from build123d import *

# Parameters (mm, degrees)
F0_W     = 35.25
F0_H     = 22.25
F1_DEPTH = 10
F2_R     = 1


with BuildPart() as f1:
    # F0 (on Top) → F1 (new body)
    with BuildSketch(Plane.XY):
        with BuildLine():
            Line((21, -9.464824), (21, 9.464824))
            ThreePointArc((21, 9.464824), (19.853951, 12.650269), (16.941176, 14.375444))
            ThreePointArc((16.941176, 14.375444), (0, 15.984287), (-16.941176, 14.375444))
            ThreePointArc((-16.941176, 14.375444), (-19.853951, 12.650269), (-21, 9.464824))
            Line((-21, 9.464824), (-21, -11.101853))
            ThreePointArc((-21, -11.101853), (-20.330458, -12.991023), (-18.62069, -14.036941))
            ThreePointArc((-18.62069, -14.036941), (-0.856643, -15.98021), (16.941176, -14.375444))
            ThreePointArc((16.941176, -14.375444), (19.853951, -12.650269), (21, -9.464824))
        make_face()
        Rectangle(F0_W, F0_H, mode=Mode.SUBTRACT)
    extrude(amount=F1_DEPTH)

    # F2
    f2_edges = [f1.edges().sort_by_distance(p)[0] for p in [
        (19.853951, 12.650269, 10),
        (19.853951, 12.650269, 0),
    ]]
    fillet(f2_edges, radius=F2_R)


solid = f1.part
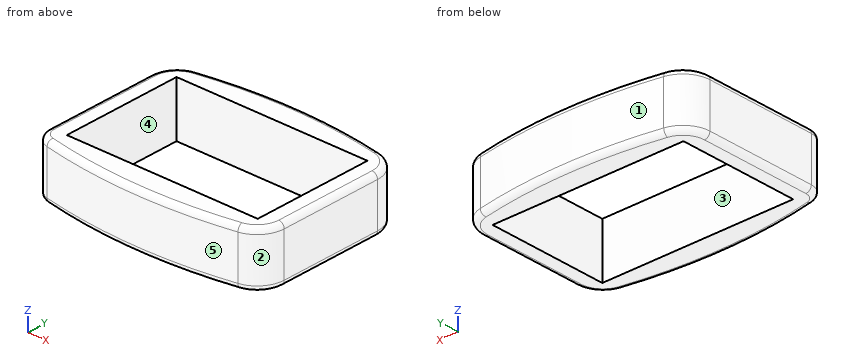
Check sheet for the modelled part. Datum: model origin and axes. Units: mm. Face numbers are marked on the shaded views. A direction names the side the tool comes from. Coordinates: 2 decimals unless noted, no trailing zeros. Write each loop counter-clockwise with the first axis right and the second up, starting at its lowest first coordinate (ties: lowest second). Pieces come first, ordered by that corner, then holes.
Item 1: Depth check by flat-ended pin: pin 1 Ø2 at (x, y) = (-11.5, -9) entering from -Z; pin 2 Ø5 at (x, z) = (8.5, 4.5) entering from -Y; pin 3 Ø1.5 at (x, z) = (-2.5, 8) entering from -Y; pin 4 Ø2 at (y, z) = (12, 4) entering from -X. Enter the tip coordinate at first touch or a pass-through.
Numbers:
pin 1: passes through
pin 2: stops at y = -15.78
pin 3: stops at y = -15.97
pin 4: stops at x = -20.76
Item 2: Scan lines: probe 1 along X at (y, z) = (-8.5, 3.5) (3 decimals); probe 2 along Y at (x, z) = (-13.5, 5.25) (3 decimals); probe 3 along Y at (x, z) = (-3, 4.75) (3 decimals). Record each from-to range of solid material in increasing order.
Numbers:
probe 1: x = -21 to -17.625, 17.625 to 21
probe 2: y = -14.966 to -11.125, 11.125 to 14.966
probe 3: y = -15.934 to -11.125, 11.125 to 15.934
Item 3: Cross-section at A-A on y = -2. Record the boundary of the cut face in (x, z) (3 decimals), then the cut area to 3 significant figures.
Numbers:
outline: (-21, 1) arc R1 ccw to (-20, 0) - (-17.625, 0) - (-17.625, 10) - (-20, 10) arc R1 ccw to (-21, 9) - close; (17.625, 0) - (20, 0) arc R1 ccw to (21, 1) - (21, 9) arc R1 ccw to (20, 10) - (17.625, 10) - close
area: 66.6 mm2
Item 4: Cross-section at B-B on z = 7.5. Record the boundary of the cut face in (x, y) (3 decimals).
Numbers:
outline: (-21, -11.102) arc R3 ccw to (-18.621, -14.037) arc R90 ccw to (16.941, -14.375) arc R5 ccw to (21, -9.465) - (21, 9.465) arc R5 ccw to (16.941, 14.375) arc R90 ccw to (-16.941, 14.375) arc R5 ccw to (-21, 9.465) - close; hole (-17.625, -11.125) - (17.625, -11.125) - (17.625, 11.125) - (-17.625, 11.125) - close
Item 5: Access from +Z, -Z, +X, -X, +Y, -Y to the whole of each face (thin tool, end or side, straight path). Record for the marked faces 4 and 5.
Numbers:
face 4: +Z, -Z
face 5: +Z, -Z, -Y
Item 6: Mould release check, pull along Y, two halves, no side actions. Record for the marked faces 1, 2 and 3: released by +Y, released by -Y, zero draft, split by the parting line, or undercut.
Numbers:
face 1: released by +Y
face 2: released by -Y
face 3: undercut
